Read the model definition and answer for the solid it produces. Units are mm, in the model's axes. A direction names the side the tool comes from. Round coordinates to 2 decimals unless told otherwise and drop trailing zeros. Loops run counter-clockwise (first coordinate to the right, second up) from the corner with the lowest first, then second, coordinate; pieces in that order, holes last. Notation, with made-up numbers: M 78.5,9 L 113.5,9 A10 ccw 113.5,16 Z; hole C -31,-24.5 d2. An arc over 180 degrees is marked long. Answer as CSV lines item,"result".
```python
from build123d import *

# Parameters (mm, degrees)
BOSS_EXTRUDE1_DEPTH = 2
BOSS_EXTRUDE2_START = -7.6
BOSS_EXTRUDE2_DEPTH = 7.6
BOSS_EXTRUDE3_DEPTH = 2
SKETCH5_W           = 38
SKETCH5_H           = 5.8
CUT_EXTRUDE1_DEPTH  = 40.954474092
SKETCH6_W           = 38
SKETCH6_H           = 3
BOSS_EXTRUDE4_DEPTH = 7.6
FILLET1_R           = 2


with BuildPart() as part:
    # Sketch1 → Boss-Extrude1 (new body)
    with BuildSketch(Plane(origin=(0, 0, 0), x_dir=(1, 0, 0), z_dir=(0, 1, 0))):
        with BuildLine():
            Line((2, 0), (36, 0))
            ThreePointArc((36, 0), (37.414213562, 0.585786438), (38, 2))
            Line((38, 2), (38, 6))
            ThreePointArc((38, 6), (37.707106781, 6.707106781), (37, 7))
            Line((37, 7), (1, 7))
            ThreePointArc((1, 7), (0.292893219, 6.707106781), (0, 6))
            Line((0, 6), (0, 2))
            ThreePointArc((0, 2), (0.585786438, 0.585786438), (2, 0))
        make_face()
    extrude(amount=BOSS_EXTRUDE1_DEPTH)

    # Sketch2 → Boss-Extrude2 (add)
    with BuildSketch(Plane(origin=(0, 2, 0), x_dir=(1, 0, 0), z_dir=(0, 1, 0)).offset(BOSS_EXTRUDE2_START)):
        with BuildLine():
            Line((38, 6), (38, 2))
            ThreePointArc((38, 2), (37.788854382, 1.105572809), (37.2, 0.4))
            Line((37.2, 0.4), (37.2, 5.3))
            ThreePointArc((37.2, 5.3), (37.053553391, 5.653553391), (36.7, 5.8))
            Line((36.7, 5.8), (1.3, 5.8))
            ThreePointArc((1.3, 5.8), (0.946446609, 5.653553391), (0.8, 5.3))
            Line((0.8, 5.3), (0.8, 0.4))
            ThreePointArc((0.8, 0.4), (0.211145618, 1.105572809), (0, 2))
            Line((0, 2), (0, 6))
            ThreePointArc((0, 6), (0.292893219, 6.707106781), (1, 7))
            Line((1, 7), (37, 7))
            ThreePointArc((37, 7), (37.707106781, 6.707106781), (38, 6))
        make_face()
    extrude(amount=BOSS_EXTRUDE2_DEPTH)

    # Sketch4 → Boss-Extrude3 (add)
    with BuildSketch(Plane.XZ.offset(5.6)):
        with BuildLine():
            Line((37, -7), (1, -7))
            ThreePointArc((1, -7), (0.292893219, -6.707106781), (0, -6))
            Line((0, -6), (0, -9))
            ThreePointArc((0, -9), (0.585786438, -10.414213562), (2, -11))
            Line((2, -11), (36, -11))
            ThreePointArc((36, -11), (37.414213562, -10.414213562), (38, -9))
            Line((38, -9), (38, -6))
            ThreePointArc((38, -6), (37.707106781, -6.707106781), (37, -7))
        make_face()
    extrude(amount=-BOSS_EXTRUDE3_DEPTH)

    # Sketch5 → Cut-Extrude1 (cut, through all)
    with BuildSketch(Plane.XZ):
        with Locations((19, -2.9)):
            Rectangle(SKETCH5_W, SKETCH5_H)
    extrude(amount=CUT_EXTRUDE1_DEPTH, mode=Mode.SUBTRACT)

    # Sketch6 → Boss-Extrude4 (add)
    with BuildSketch(Plane.XZ.offset(5.6)):
        with Locations((19, -5.5)):
            Rectangle(SKETCH6_W, SKETCH6_H)
    extrude(amount=-BOSS_EXTRUDE4_DEPTH)

    # Fillet1
    fillet1_edges = [part.edges().sort_by_distance(p)[0] for p in [
        (19, 2, -7),
        (19, -3.6, -7),
    ]]
    fillet(fillet1_edges, radius=FILLET1_R)


solid = part.part
```
1) Find section A-A, the plane x = 10. Give the vertices of the cut face in (y, z), then the cut area to 3 significant figures.
Evaluation:
outline,"M -5.6,-11 L -3.6,-11 L -3.6,-9 A2 cw -1.6,-7 L 0,-7 A2 ccw 2,-5 L 2,0 L 0,0 L 0,-4 L -5.6,-4 Z"
area,"38.8 mm^2"
2) Find section D-D, the plane y = -1. Give the vertices of the cut face in (x, z), then the cut area to 3 significant figures.
Evaluation:
outline,"M 0,-7 L 38,-7 L 38,-4 L 0,-4 Z"
area,"114 mm^2"
3) A tool of negligible diameter and unlimited length cuts with its end or side. For faces 1 (the cylindrical face through (37.4, 0.99, -0.57)), 2 (the flat face through (19, -3, -4)), 3 (the flat face through (19, -3.6, -10)), from which of +Z, -Z, +X, -X, +Y, -Y can it reach the whole face along a straight path? Write none if from no direction.
Evaluation:
face 1,"+Z, +X, +Y, -Y"
face 2,"+Z, +X, -X, -Y"
face 3,"-Z, +X, -X, +Y"
4) Determine the mould class of faces 4 (the cylindrical face through (37.4, -4.61, -10.43)), 5 (the cylindrical face through (0.57, -4.61, -10.4)), 6 (the flat face through (19, -1, -7)) for opening direction X: released by +X, released by -X, zero draft, split by the parting line, or undercut.
Evaluation:
face 4,"released by +X"
face 5,"released by -X"
face 6,"zero draft"
5) Each of these flat-tipped pins is pushed along its axis until it touches: P1, Ø2, axis at x = 27.5, z = -2.5, coming from the -Y side; P2, Ø1.7, axis at x = 20, y = -3.5, coming from the +Z side; P3, Ø1, axis at x = 24.5, z = -10.5, coming from the +Y side; P4, Ø3, axis at y = 0.5, z = -9, coming from the +X side. Where does it stop, or does it pass through?
Evaluation:
P1,"stops at y = 0"
P2,"stops at z = -4"
P3,"stops at y = -3.6"
P4,"passes through"
6) Find section B-B, the plane y = -4.25. Give the vertices of the cut face in (x, z).
Evaluation:
outline,"M 0,-9 A2 ccw 2,-11 L 36,-11 A2 ccw 38,-9 L 38,-4 L 0,-4 Z"
7) Straight lines are drawn through the part: line 1 (Y direction, x = 2.5, z = -3.25); line 2 (Z direction, x = 9.5, y = -1.25); line 3 (Z direction, x = 31.5, y = -5). For each, find the intervals that lie inside material, in ascending order.
Evaluation:
line 1,"y = 0 to 2"
line 2,"z = -7 to -4"
line 3,"z = -11 to -4"
8) Find section C-C, the plane z = -3. Give the vertices of the cut face in (x, y), then the cut area to 3 significant figures.
Evaluation:
outline,"M 0,0 L 38,0 L 38,2 L 0,2 Z"
area,"76.0 mm^2"
